Source: CAD feature listing. Evaluate the final solid. Frame: model axes, mm. A direction names the side the tool comes from. Coordinates: 2 decimals unless noted, no trailing zeros. Write each loop counter-clockwise with the first axis right and the second up, starting at its lowest first coordinate (ties: lowest second). Pieces come first, ordered by that corner, then holes. Notation, with made-up numbers: M 72,74.25 L 81,74.25 A21 cw 81,85.25 Z; hole C 84.25,80.25 d5. An arc over 180 degrees is marked long. One line per item, written item: value. Start each with the question number.
Item 1: Mould query, pull axis X, two halves, no side actions, for faces 4 (the cylindrical face through (-23.859, 4.93, -23.797)), 5 (the cylindrical face through (10.743, 0.493, 6.39)), 6 (the flat face through (0, 0, 0)). Classes: released by +X, released by -X, zero draft, split by the parting line, or undercut.
Item 2: Cut plane B-B, the plane z = -20. State how many separate pieces and enclosed holes the cut face has, then the cut area to 3 significant figures.
Item 3: Cut plane A-A, the plane y = 5.5. Output: boundary loops of the cut face in (x, z).
Item 4: Set-up query: faces 1 (the flat face through (25, 5, 0)), 2 (the cylindrical face through (-22.44, 8.52, 21.27)), 3 (the cylindrical face through (-10.906, 0.493, 6.109)). Return all of +Z, -Z, +X, -X, +Y, -Y with unobstructed straight access to the full face (end or side cutting, diameter ignored); none if empty.
Item 5: Ray query, L1, parallel to Z at x = 4, y = 8; L2, parallel to Z at x = 20, y = 7.8; L3, parallel to Z at x = 8, y = 0.5. Return the intervals inside material, ascending. Write a range as from..to.
Item 6: Pin query (flat end, axial travel): P1, Ø4.5, axis at x = 20, z = -21, coming from the +Y side; P2, Ø8, axis at x = 6.5, z = -4, coming from the +Y side; P3, Ø3, axis at x = -19.5, z = 19, coming from the +Y side. Return the tip coordinate at first contact, or that it passes through.
```python
from build123d import *

# Parameters (mm, degrees)
SKETCH1_W           = 50
SKETCH1_H           = 50
SKETCH1_R           = 24
BOSS_EXTRUDE1_DEPTH = 10
CHAMFER1_SIZE       = 3
BOSS_EXTRUDE2_START = -2.999999
SKETCH4_W           = 50
SKETCH4_H           = 50
SKETCH4_W_2         = 48
SKETCH4_H_2         = 48
BOSS_EXTRUDE2_DEPTH = 2.999999
SKETCH5_R           = 2.75
CUT_EXTRUDE1_DEPTH  = 3
FILLET1_R           = 4
SKETCH6_R           = 12.5
BOSS_EXTRUDE5_DEPTH = 1
SKETCH7_R           = 2.15
CUT_EXTRUDE2_DEPTH  = 21
SKETCH9_W           = 3
SKETCH9_H           = 24
BOSS_EXTRUDE6_DEPTH = 1
CIRPATTERN1_COUNT   = 3


with BuildPart() as part:
    # Sketch1 → Boss-Extrude1 (new body)
    with BuildSketch(Plane(origin=(0, 0, 0), x_dir=(1, 0, 0), z_dir=(0, 1, 0))):
        Rectangle(SKETCH1_W, SKETCH1_H)
        with Locations(Location((0, 0, 0), (0, 0, 270))):
            Circle(SKETCH1_R, mode=Mode.SUBTRACT)
    extrude(amount=BOSS_EXTRUDE1_DEPTH)

    # Chamfer1
    # the kernel refuses this chamfer: 3 mm, written as the material it takes off along each edge
    with BuildSketch(Plane(origin=(0, 10, 0), x_dir=(0, 0, 1), z_dir=(-1, 0, 0))) as chamfer1_piece_1:
        Polygon((24, -CHAMFER1_SIZE), (24 + CHAMFER1_SIZE, 0), (24, 0), align=None)
    revolve(axis=Axis((0, 10, 0), (0, 1, 0)), mode=Mode.SUBTRACT)

    # Sketch4 → Boss-Extrude2 (add)
    with BuildSketch(Plane(origin=(0, 10, 0), x_dir=(1, 0, 0), z_dir=(0, 1, 0)).offset(BOSS_EXTRUDE2_START)):
        Rectangle(SKETCH4_W, SKETCH4_H)
        Rectangle(SKETCH4_W_2, SKETCH4_H_2, mode=Mode.SUBTRACT)
    extrude(amount=BOSS_EXTRUDE2_DEPTH)

    # Sketch5 → Cut-Extrude1 (cut)
    with BuildSketch(Plane(origin=(0, 10, 0), x_dir=(1, 0, 0), z_dir=(0, 1, 0))):
        with Locations(Location((-20, 20, 0), (0, 0, 270))):
            Circle(SKETCH5_R)
        with Locations(Location((20, 20, 0), (0, 0, 270))):
            Circle(SKETCH5_R)
        with Locations(Location((20, -20, 0), (0, 0, 270))):
            Circle(SKETCH5_R)
        with Locations(Location((-20, -20, 0), (0, 0, 270))):
            Circle(SKETCH5_R)
    extrude(amount=-CUT_EXTRUDE1_DEPTH, mode=Mode.SUBTRACT)

    # Fillet1
    fillet1_edges = [part.edges().sort_by_distance(p)[0] for p in [
        (-25, 5, -25),
        (25, 5, -25),
        (25, 5, 25),
        (-25, 5, 25),
    ]]
    fillet(fillet1_edges, radius=FILLET1_R)

    # Sketch7 → Cut-Extrude2 (cut)
    with BuildSketch(Plane(origin=(0, 7, 0), x_dir=(1, 0, 0), z_dir=(0, 1, 0))):
        with Locations(Location((-20, -20, 0), (0, 0, 270))):
            Circle(SKETCH7_R)
        with Locations(Location((-20, 20, 0), (0, 0, 270))):
            Circle(SKETCH7_R)
        with Locations(Location((20, 20, 0), (0, 0, 270))):
            Circle(SKETCH7_R)
        with Locations(Location((20, -20, 0), (0, 0, 270))):
            Circle(SKETCH7_R)
    extrude(amount=-CUT_EXTRUDE2_DEPTH, mode=Mode.SUBTRACT)



with BuildPart() as body_2:
    # Sketch6 → Boss-Extrude5 (new body)
    with BuildSketch(Plane(origin=(0, 0, 0), x_dir=(1, 0, 0), z_dir=(0, 1, 0))):
        with Locations(Location((0, 0, 0), (0, 0, 270))):
            Circle(SKETCH6_R)
    extrude(amount=BOSS_EXTRUDE5_DEPTH)


with BuildPart() as part_1:
    add(part.part)

    add(body_2.part)  # Boss-Extrude6 merges body 2
    # Sketch9 → Boss-Extrude6 (add)
    with BuildSketch(Plane.XZ):
        with Locations((0, 12.5)):
            Rectangle(SKETCH9_W, SKETCH9_H)
    boss_extrude6 = extrude(amount=-BOSS_EXTRUDE6_DEPTH)

    # CirPattern1: Boss-Extrude6 ×3 about axis
    cirpattern1_axis = Axis((0, 0, 0), (0, 1, 0))
    for i in range(1, CIRPATTERN1_COUNT):
        add(boss_extrude6.rotate(cirpattern1_axis, i * 360 / CIRPATTERN1_COUNT))


solid = part_1.part
```
From the geometry:
1. face 4: released by -X
1. face 5: undercut
1. face 6: zero draft
2. separate pieces: 4
2. enclosed holes: 0
2. area: 127 mm²
3. outline: M -25,-21 A4 ccw -21,-25 L 21,-25 A4 ccw 25,-21 L 25,21 A4 ccw 21,25 L -21,25 A4 ccw -25,21 Z; hole C 0,0 d48; hole C -20,-20 d4.3; hole C -20,20 d4.3; hole C 20,-20 d4.3; hole C 20,20 d4.3
4. face 1: +Z, -Z, +X, +Y, -Y
4. face 2: +Y
4. face 3: +Y, -Y
5. L1: z = -25..-24, 24..25
5. L2: z = -25..-22.75, -17.25..-14.66, 14.66..17.25, 22.75..25
5. L3: z = -25..-22.63, -9.6..9.6, 22.63..25
6. P1: stops at y = 10
6. P2: stops at y = 1
6. P3: stops at y = 7
